from build123d import *

# Parameters (mm, degrees)
SKETCH1_R           = 15.748
BOSS_EXTRUDE1_DEPTH = 6.35
SKETCH2_R           = 1.4224
SKETCH2_R_2         = 1.03251
CUT_EXTRUDE1_DEPTH  = 6.35


with BuildPart() as part:
    # Sketch1 → Boss-Extrude1 (new body)
    with BuildSketch(Plane(origin=(0, 0, 0), x_dir=(0, 0, -1), z_dir=(1, 0, 0))):
        Polygon((0, 0), (70, 0), (70, 49.756615014), (64.872483647, 54.884131367), (70, 60.011647719), (70, 70), (60.148635267, 70), (54.952625141, 64.803989874), (49.756615014, 70), (0, 70), align=None)
        with Locations((35, 35)):
            Circle(SKETCH1_R, mode=Mode.SUBTRACT)
    extrude(amount=BOSS_EXTRUDE1_DEPTH)

    # Sketch2 → Cut-Extrude1 (cut)
    with BuildSketch(Plane(origin=(6.35, 0, 0), x_dir=(0, 0, -1), z_dir=(1, 0, 0))):
        with Locations((8.75, 61.25)):
            Circle(SKETCH2_R)
        with Locations((8.75, 8.75)):
            Circle(SKETCH2_R_2)
        with Locations((61.25, 8.75)):
            Circle(SKETCH2_R_2)
    extrude(amount=-CUT_EXTRUDE1_DEPTH, mode=Mode.SUBTRACT)


solid = part.part
Read the model definition and answer for the solid it produces. Units are mm, in the model's axes. A direction names the side the tool comes from. Round coordinates to 2 decimals unless told otherwise and drop trailing zeros. Loops run counter-clockwise (first coordinate to the right, second up) from the corner with the lowest first, then second, coordinate; pieces in that order, holes last. Notation, with made-up numbers: (71.25, 20.5) - (118.25, 20.5) arc R27 ccw to (118.25, 56.5) - close; hole circle Ø2 at (5, 16). An arc over 180 degrees is marked (long way). One line per question, with ' | ' between items. Start each with the question number.
Q1. For faces 4 (the flat face through (3.13, 57.41, -67.4)), 5 (the cylindrical face through (3.131, 48.279, -43.466)), 6 (the flat face through (3.13, 67.44, -57.59)), determine the directions among +Z, -Z, +X, -X, +Y, -Y from which every point of the face is accessible in a straight line to the end or side of a thin tool.
Q2. For a pull along Z with two mould halves and no side action, classify faces 1 (the cylindrical face through (3.219, 9.621, -9.305)), 2 (the flat face through (3, 0, -35)), 3 (the flat face through (3.131, 52.284, -67.472)) as +Z half, -Z half, draft (parallel to the pull), parting line (faces both ways), or undercut.
Q3. Section C-C on y = 61.25 is taken. Give the vertices of the cut face in (x, z), plus the area to 3 significant figures.
Q4. Section B-B on z = -8.75 is taken. Give the vertices of the cut face in (x, y), plus the area to 3 significant figures.
Q5. Find the intervals of material crossed by L1, parallel to Y at x = 2.5, z = -8.75; L2, parallel to Z at x = 3.5, y = 37; L3, parallel to Z at x = 6.25, y = 31, in increasing order.
Q6. Flat-ended cylindrical pins translate along their axes: pin 1 (1.5 mm diameter, centred on x = 4, z = -42.5, fed in from -Y); pin 2 (19 mm diameter, centred on y = 35, z = -35, fed in from -X). Find the tip coordinate at first contact, or state that the pin passes through.
Q7. Section D-D on x = 2.5 is taken. Give the vertices of the cut face in (y, z), plus the area to 3 significant figures.
Q8. Section A-A on z = -61.25 is taken. Give the vertices of the cut face in (x, y).
Established:
1) face 4: -Z, +X, -X | face 5: +X, -X | face 6: +X, -X, +Y
2) face 1: undercut | face 2: draft | face 3: -Z half
3) outline: (0, -70) - (6.35, -70) - (6.35, -10.17) - (0, -10.17) - close; (0, -7.33) - (6.35, -7.33) - (6.35, 0) - (0, 0) - close | area: 426 mm²
4) outline: (0, 0) - (6.35, 0) - (6.35, 7.72) - (0, 7.72) - close; (0, 9.78) - (6.35, 9.78) - (6.35, 59.83) - (0, 59.83) - close; (0, 62.67) - (6.35, 62.67) - (6.35, 70) - (0, 70) - close | area: 413 mm²
5) L1: 0 to 7.72, 9.78 to 59.83, 62.67 to 70 | L2: -70 to -50.62, -19.38 to 0 | L3: -70 to -50.23, -19.77 to 0
6) pin 1: y = 0 | pin 2: through
7) outline: (0, -70) - (49.76, -70) - (54.88, -64.87) - (60.01, -70) - (70, -70) - (70, -60.15) - (64.8, -54.95) - (70, -49.76) - (70, 0) - (0, 0) - close; hole circle Ø2.07 at (8.75, -61.25); hole circle Ø2.07 at (8.75, -8.75); hole circle Ø31.5 at (35, -35); hole circle Ø2.84 at (61.25, -8.75) | area: 4,050 mm²
8) outline: (0, 0) - (6.35, 0) - (6.35, 7.72) - (0, 7.72) - close; (0, 9.78) - (6.35, 9.78) - (6.35, 70) - (0, 70) - close
